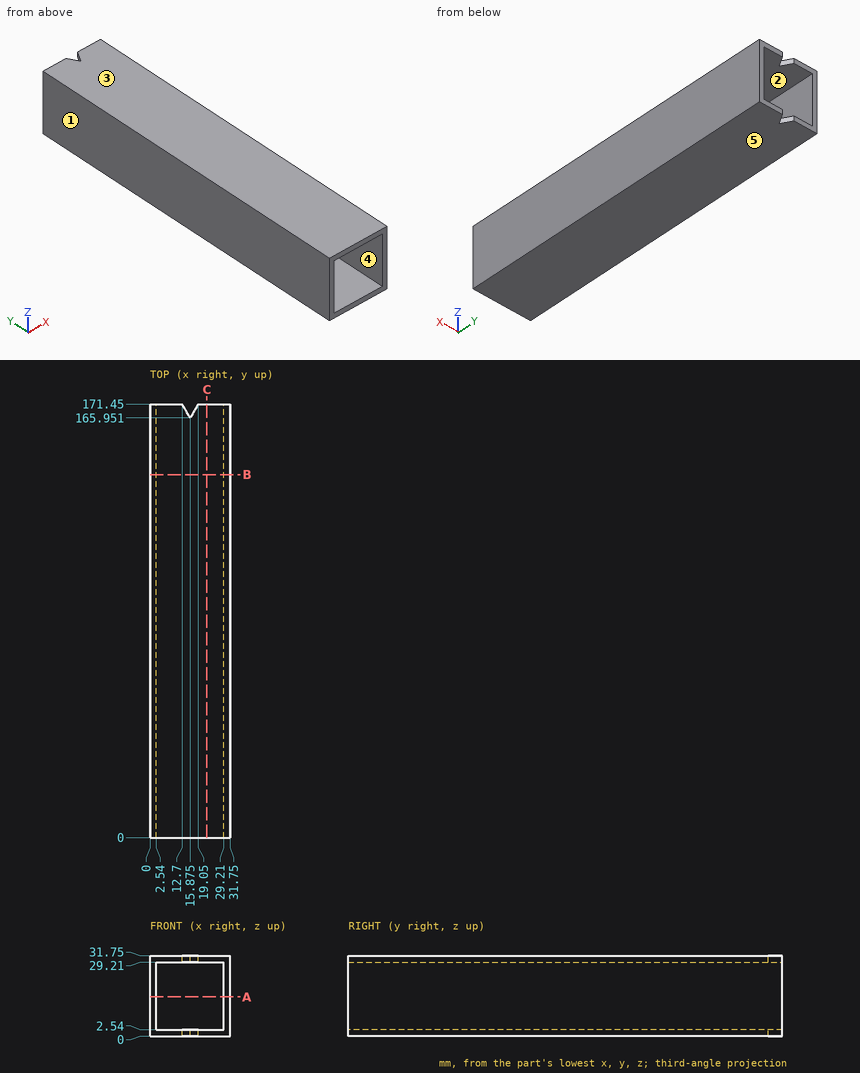
Job drawing, mm, ordinate dimensions from the low corner. One solid piece. A direction names the side the tool comes from. Give positions to 0.01 mm unless a question says otherwise; leave off trailing zeros. Loops run counter-clockwise (first coordinate to the right, second up) from the corner with the lowest first, then second, coordinate; pieces in that order, holes last. Notation, with made-up numbers: (60.5, -2.75) -> (64.5, -2.75) arc R21 cw to (64.5, 28.25) -> close; hole circle Ø8 at (64, 72.25). An arc over 180 degrees is marked (long way). Use a Markdown table: item, result. Add a question column.
(1) Slice it at C-C on x = 22.5. List the corners of the cut face in (y, z), and give its area (3 significant figures).
(2) Mould opens along X. For the marked faces 1, 2 and 3 say: +X half, -X half, draft (parallel to the pull), parting line (faces both ways), or undercut.
(3) Slice it at B-B on y = 143.5. List the corners of the cut face in (x, z), and give its area (3 significant figures).
(4) Tool access for the marked faces 4 and 5: list every direction of +Z, -Z, +X, -X, +Y, -Y with a clear straight run to the whole face (end or side of a thin tool).
(5) Wall check: line 1 along Z through (x, y) = (19, 89). Give the ranges that are in metal, low to high.
(6) Drop a flat-ended pin along its axis: pin 1 Ø5 at (y, z) = (94.5, 12) entering from -X. Give the stop position or say it passes through.
(7) Slice it at A-A on z = 15.5. List the corners of the cut face in (x, y).
Filled sheet:
| question | item | result |
|---|---|---|
| 1 | outline | (0, 0) -> (171.45, 0) -> (171.45, 2.54) -> (0, 2.54) -> close; (0, 29.21) -> (171.45, 29.21) -> (171.45, 31.75) -> (0, 31.75) -> close |
| 1 | area | 871 mm2 |
| 2 | face 1 | -X half |
| 2 | face 2 | undercut |
| 2 | face 3 | draft |
| 3 | outline | (0, 0) -> (31.75, 0) -> (31.75, 31.75) -> (0, 31.75) -> close; hole (2.54, 2.54) -> (29.21, 2.54) -> (29.21, 29.21) -> (2.54, 29.21) -> close |
| 3 | area | 297 mm2 |
| 4 | face 4 | +Y, -Y |
| 4 | face 5 | -Z, +X, -X, +Y, -Y |
| 5 | line 1 | 0 to 2.54, 29.21 to 31.75 |
| 6 | pin 1 | x = 0 |
| 7 | outline | (0, 0) -> (2.54, 0) -> (2.54, 171.45) -> (0, 171.45) -> close; (29.21, 0) -> (31.75, 0) -> (31.75, 171.45) -> (29.21, 171.45) -> close |
